Here's how the part is built. I have some questions about the finished solid (model axes, mm). A direction names the side the tool comes from. Coordinates: 2 decimals unless noted, no trailing zeros. Write each loop counter-clockwise with the first axis right and the second up, starting at its lowest first coordinate (ties: lowest second). Pieces come first, ordered by that corner, then holes. Notation, with made-up numbers: (80, 22) - (113, 22) arc R22 cw to (113, 39) - close; hole circle Ø4 at (55.25, 55). An arc over 180 degrees is marked (long way). Answer in a Markdown table with one row per item. Add a question column.
Item 1: Imagine slicing it at B-B (z = 16). Please give me the cut outline in (x, y).
Item 2: Imagine slicing it at A-A (x = 0). Please give me the cut outline in (y, z), plus the area to 3 significant figures.
Item 3: If I drill on probe 1 along X at (y, z) = (20, 17); probe 2 along Y at (x, z) = (150, 30); probe 3 along X at (y, z) = (16.5, 14.5), over which ranges is the centre line in solid material (lowest first)? Write a range as from..to.
Item 4: I'm going to push flat-ended pins straight in: pin 1 (6 mm diameter, centred on x = -67.5, y = -34.5, fed in from -Z); pin 2 (12 mm diameter, centred on x = 104, z = 10, fed in from -Y); pin 3 (1.7 mm diameter, centred on x = 139.5, y = 38, fed in from -Z); pin 4 (3 mm diameter, centred on y = -38, z = 72, fed in from +X). Where does each tip first touch, or does it pass through?
Item 5: Imagine slicing it at D-D (z = 46.5). Please give me the cut outline in (x, y).
Item 6: Imagine slicing it at C-C (y = 10). Please give me the cut outline in (x, z), plus the area to 3 significant figures.
Item 7: Which directions (+Z, -Z, +X, -X, +Y, -Y) give clear straight access to the entire face, cutting with the end or side of a thin tool? Please do faces 1 (the face through (-189.96, 1.76, 36.25)), 2 (the face through (149, -26, 60)), 3 (the face through (-95.68, -34.63, 19.72)), 4 (the face through (-94.13, 34.92, 19.72)).
from build123d import *

# Parameters (mm, degrees)
SKETCH1_R           = 25
SKETCH1_R_2         = 25.531825786
BOSS_EXTRUDE1_DEPTH = 40
SKETCH2_R           = 40
SKETCH2_R_2         = 25
SKETCH2_R_3         = 25.531825786
BOSS_EXTRUDE2_DEPTH = 20
SKETCH3_R           = 60
SKETCH3_R_2         = 50
BOSS_EXTRUDE3_DEPTH = 50
SKETCH4_R           = 50
CUT_EXTRUDE1_DEPTH  = 50


with BuildPart() as part:
    # Sketch1 → Boss-Extrude1 (new body)
    with BuildSketch(Plane.XY):
        with BuildLine():
            ThreePointArc((-150, -40), (-94.903714286, -34.773015604), (-45.465365878, -59.648139163))
            ThreePointArc((-45.465365878, -59.648139163), (5.116377771, -74.825281012), (53.161436396, -52.904269017))
            ThreePointArc((53.161436396, -52.904269017), (99.897642557, -33.821692035), (150, -40))
            ThreePointArc((150, -40), (190, 0), (150, 40))
            ThreePointArc((150, 40), (99.897642557, 33.821692035), (53.161436396, 52.904269017))
            ThreePointArc((53.161436396, 52.904269017), (5.116377771, 74.825281012), (-45.465365878, 59.648139163))
            ThreePointArc((-45.465365878, 59.648139163), (-94.903714286, 34.773015604), (-150, 40))
            ThreePointArc((-150, 40), (-190, 0), (-150, -40))
        make_face()
        with Locations((-150, 0)):
            Circle(SKETCH1_R, mode=Mode.SUBTRACT)
        with Locations((150, 0)):
            Circle(SKETCH1_R_2, mode=Mode.SUBTRACT)
    extrude(amount=BOSS_EXTRUDE1_DEPTH)

    # Sketch2 → Boss-Extrude2 (add)
    with BuildSketch(Plane.XY.offset(40)):
        with Locations((-150, 0)):
            Circle(SKETCH2_R)
        with Locations((-150, 0)):
            Circle(SKETCH2_R_2, mode=Mode.SUBTRACT)
        with Locations((150, 0)):
            Circle(SKETCH2_R)
        with Locations((150, 0)):
            Circle(SKETCH2_R_3, mode=Mode.SUBTRACT)
    extrude(amount=BOSS_EXTRUDE2_DEPTH)

    # Sketch3 → Boss-Extrude3 (add)
    with BuildSketch(Plane.XY.offset(40)):
        Circle(SKETCH3_R)
        Circle(SKETCH3_R_2, mode=Mode.SUBTRACT)
    extrude(amount=BOSS_EXTRUDE3_DEPTH)

    # Sketch4 → Cut-Extrude1 (cut)
    with BuildSketch(Plane.XY.offset(40)):
        Circle(SKETCH4_R)
    extrude(amount=-CUT_EXTRUDE1_DEPTH, mode=Mode.SUBTRACT)


solid = part.part
Here are the results:
| question | item | result |
|---|---|---|
| 1 | outline | (-150, -40) arc R100 cw to (-45.47, -59.65) arc R75 ccw to (53.16, -52.9) arc R100 cw to (150, -40) arc R40 ccw to (150, 40) arc R100 cw to (53.16, 52.9) arc R75 ccw to (-45.47, 59.65) arc R100 cw to (-150, 40) arc R40 ccw to start; hole circle Ø50 at (-150, 0); hole circle Ø100 at (0, 0); hole circle Ø51.06 at (150, 0) |
| 2 | outline | (-75, 0) - (-50, 0) - (-50, 90) - (-60, 90) - (-60, 40) - (-75, 40) - close; (50, 0) - (75, 0) - (75, 40) - (60, 40) - (60, 90) - (50, 90) - close |
| 2 | area | 3,000 mm2 |
| 3 | probe 1 | x = -184.64..-165, -135..-45.83, 45.83..134.13, 165.87..184.64 |
| 3 | probe 2 | y = -40..-25.53, 25.53..40 |
| 3 | probe 3 | x = -186.44..-168.78, -131.22..-47.2, 47.2..130.52, 169.48..186.44 |
| 4 | pin 1 | stops at z = 0 |
| 4 | pin 2 | stops at y = -34.09 |
| 4 | pin 3 | stops at z = 40 |
| 4 | pin 4 | stops at x = 47.62 |
| 5 | outline | circle Ø80 at (-150, 0); circle Ø120 at (0, 0); circle Ø80 at (150, 0); hole circle Ø50 at (-150, 0); hole circle Ø100 at (0, 0); hole circle Ø51.06 at (150, 0) |
| 6 | outline | (-188.73, 0) - (-172.91, 0) - (-172.91, 60) - (-188.73, 60) - close; (-127.09, 0) - (-48.99, 0) - (-48.99, 90) - (-59.16, 90) - (-59.16, 40) - (-111.27, 40) - (-111.27, 60) - (-127.09, 60) - close; (48.99, 0) - (126.51, 0) - (126.51, 60) - (111.27, 60) - (111.27, 40) - (59.16, 40) - (59.16, 90) - (48.99, 90) - close; (173.49, 0) - (188.73, 0) - (188.73, 60) - (173.49, 60) - close |
| 6 | area | 9,730 mm2 |
| 7 | face 1 | +Z |
| 7 | face 2 | +Z, +X, +Y, -Y |
| 7 | face 3 | -Z, -Y |
| 7 | face 4 | -Z, +Y |
